from build123d import *

# Parameters (mm, degrees)
F0_R           = 100
F1_DEPTH       = 30
F2_R           = 40
F3_DEPTH       = 129.3
F4_R           = 14.99999
F6_D           = 45
F6_DEPTH       = 200
F6_CBORE_D     = 65
F6_CBORE_DEPTH = 80
F6_TIP         = 13.5193639281


# Not quite as in the source:
# - a fillet or chamfer is up to 0.001 mm smaller than in the source, because OpenCascade refuses the exact size


with BuildPart() as f1:
    # F0 (on Top) → F1 (new body)
    with BuildSketch(Plane.XY):
        Circle(F0_R)
    extrude(amount=F1_DEPTH)

    # F2 (on face) → F3 (join, symmetric)
    with BuildSketch(Plane.XY.offset(30)):
        Circle(F2_R)
    extrude(amount=F3_DEPTH, both=True)

    # F4 (radius 15 in the source; OpenCascade refuses exactly that, so slightly less here)
    f4_edges = [f1.edges().sort_by_distance(p)[0] for p in [
        (-100, 0, 30),
        (100, 0, 15),
        (-100, 0, 0),
    ]]
    fillet(f4_edges, radius=F4_R)

    # F6
    with Locations(Plane.XY.offset(159.3)):
        with Locations((0, 0)):
            CounterBoreHole(F6_D / 2, F6_CBORE_D / 2, F6_CBORE_DEPTH, depth=F6_DEPTH)
            with Locations((0, 0, -(F6_DEPTH + F6_TIP / 2))):  # 118° drill point
                Cone(0, F6_D / 2, F6_TIP, mode=Mode.SUBTRACT)


solid = f1.part
For this review, take the finished solid that the model builds, in its own axes (mm). A direction names the side the tool comes from. Coordinates: 2 decimals unless noted, no trailing zeros. Order: outer loops, then holes, each group sorted by start corner. A loop starts at its lowest first (then second) coordinate and runs counter-clockwise, first axis right, second up. Notation, with made-up numbers: (-10, 27) - (16, 27) arc R22 cw to (16, 59) - close; hole circle Ø6 at (55.5, 29.25). An arc over 180 degrees is marked (long way). Use one line per item in the form item = value.
Q1. Consider section B-B (z = 45). Give the boundary of the cut face in (x, y), then the cut area to 3 significant figures.
Checked values:
outline = circle Ø80 at (0, 0); hole circle Ø45 at (0, 0)
area = 3,440 mm2
Q2. For faces 5 (the flat face through (0, 33, 159.3)), 6 (the flat face through (37, -18, 0)), 7 (the cylindrical face through (-10.382, -19.961, 18.46)), list the 3-axis set-ups (+Z, -Z, +X, -X, +Y, -Y) from which the entire face can be reached by the end or side of a thin tool; tool diameter is ignored.
Checked values:
face_5 = +Z, +X, -X, +Y, -Y
face_6 = -Z
face_7 = +Z
Q3. For probe 1 along Y at (x, z) = (0, 39.5); probe 2 along Z at (x, y) = (-65.5, 40.5); probe 3 along X at (y, z) = (19, 5), list the stretches that pass through material, from the lowest coordinate up. Write a range as from..to.
Checked values:
probe_1 = -40..-22.5, 22.5..40
probe_2 = 0..30
probe_3 = -94.28..-12.05, 12.05..94.28
Q4. Consider section A-A (z = 97). Give the boundary of the cut face in (x, y).
Checked values:
outline = circle Ø80 at (0, 0); hole circle Ø65 at (0, 0)
Q5. For P1, Ø8, axis at x = 31, y = -62, coming from the -Z side; P2, Ø6, axis at x = 0, z = 49, coming from the +Y side; P3, Ø1.5, axis at x = 19.5, z = -23, coming from the -Y side, all flat-tipped, find the tip position at first contact; note any pin that passes through.
Checked values:
P1 = 0
P2 = 40
P3 = -35.33
Q6. Draft analysis for pull direction X (two halves, no side actions). For faces 1 (the cylindrical face through (31, 9.76, 119.86)), 2 (the flat face through (-1, 1, -99.3)), 3 (the flat face through (7, 22, 79.3)), 4 (the cylindrical face through (-8.67, -39.05, 95.56)), state which applies: +X half, -X half, draft (parallel to the pull), parting line (faces both ways), or undercut.
Checked values:
face_1 = undercut
face_2 = draft
face_3 = undercut
face_4 = parting line
